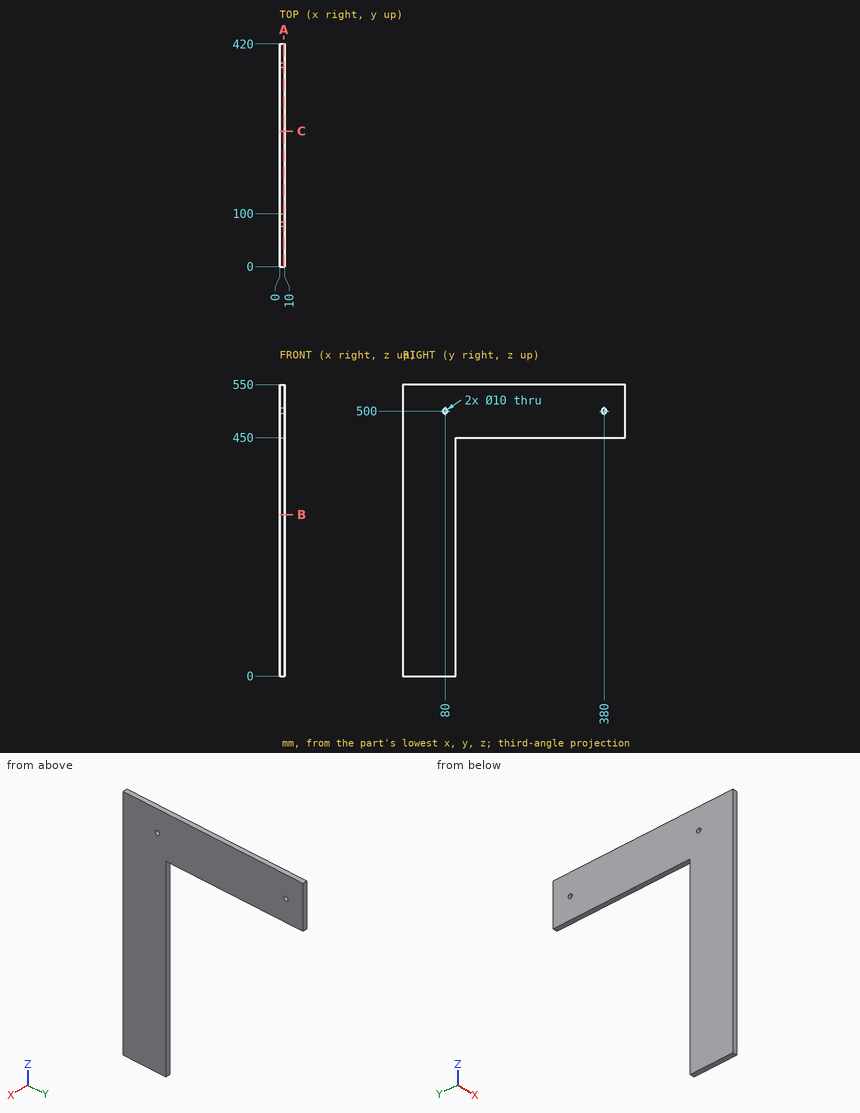
Design review of the part shown in the three views and the two pictorial views. Dimensions are in mm from the part's minimum x, y and z. Round coordinates to 2 decimals unless told otherwise and drop trailing zeros. Loops run counter-clockwise (first coordinate to the right, second up) from the corner with the lowest first, then second, coordinate; pieces in that order, holes last. Notation, with made-up numbers: (69, 42) - (75, 42) arc R20 cw to (75, 57) - close; hole circle Ø7 at (17, -8). An arc over 180 degrees is marked (long way). Use CSV: the item, a comma, the result in double quotes.
(1) Take a section at C-C, the plane y = 255.5. Give the boundary of the cut face in (x, z), plus the area to 3 significant figures.
Working result:
outline,"(0, 450) - (10, 450) - (10, 550) - (0, 550) - close"
area,"1,000 mm^2"
(2) Take a section at B-B, the plane z = 304.5. Give the boundary of the cut face in (x, y), plus the area to 3 significant figures.
Working result:
outline,"(0, 0) - (10, 0) - (10, 100) - (0, 100) - close"
area,"1,000 mm^2"
(3) Take a section at A-A, the plane x = 8.25. Give the boundary of the cut face in (y, z), plus the area to 3 significant figures.
Working result:
outline,"(0, 0) - (100, 0) - (100, 450) - (420, 450) - (420, 550) - (0, 550) - close; hole circle Ø10 at (80, 500); hole circle Ø10 at (380, 500)"
area,"86,800 mm^2"
(4) For line 1 (Y direction, x = 7.25, z = 500); line 2 (Z direction, x = 7.5, y = 380); line 3 (Y direction, x = 2.25, z = 440.5), list the stretches that pass through material, from the lowest coordinate up.
Working result:
line 1,"y = 0 to 75, 85 to 375, 385 to 420"
line 2,"z = 450 to 495, 505 to 550"
line 3,"y = 0 to 100"
(5) Clearance check with flat-ended pins moving along their axes: P1, Ø16, axis at y = 380, z = 500, coming from the +X side; P2, Ø4, axis at x = 8, y = 251.5, coming from the -Z side; P3, Ø3, axis at x = 4, z = 154.5, coming from the +Y side. State where each tip first meets the part, or that it passes through.
Working result:
P1,"stops at x = 10"
P2,"stops at z = 450"
P3,"stops at y = 100"
